Check sheet for the modelled part. Datum: model origin and axes. Units: mm. Face numbers are marked on the shaded views. A direction names the side the tool comes from. Round coordinates to 2 decimals unless told otherwise and drop trailing zeros. Loops run counter-clockwise (first coordinate to the right, second up) from the corner with the lowest first, then second, coordinate; pieces in that order, holes last. Notation, with made-up numbers: (-20, 34.5) -> (1, 34.5) arc R21 cw to (1, 73.5) -> close; hole circle Ø2 at (69, -10.75). An arc over 180 degrees is marked (long way). Return JSON: item names as keys, results as strings.
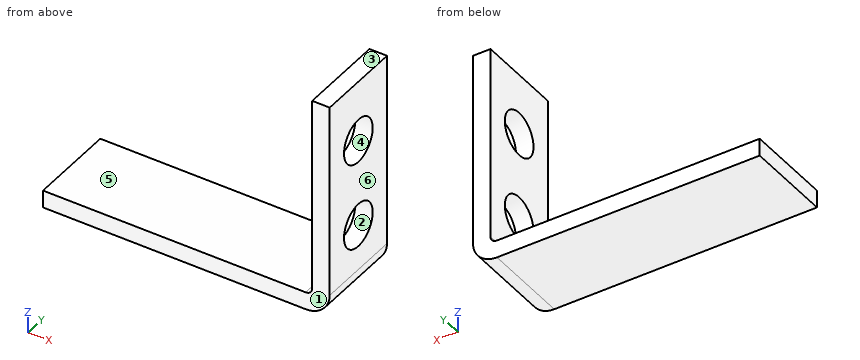
from build123d import *

# Parameters (mm, degrees)
SKETCH2_W          = 30
SKETCH2_H          = 10
BASE_FLANGE1_DEPTH = 2
EDGE_FLANGE1_DEPTH = 10
SKETCH10_R         = 2.5
CUT_EXTRUDE1_DEPTH = 39.713545169


# Sheet-metal steps are written as plain solids
with BuildPart() as part:
    # Sketch2 → Base-Flange1 (new body)
    with BuildSketch(Plane.XY):
        Rectangle(SKETCH2_W, SKETCH2_H)
    extrude(amount=-BASE_FLANGE1_DEPTH)

    # Edge-Flange1 section (across the edge) → Edge-Flange1 (add)
    with BuildSketch(Plane(origin=(15.7366, -5, 0), x_dir=(-1, 0, 0), z_dir=(0, 1, 0))):
        with BuildLine():
            Line((-2, 0.7366), (-2, 23))
            Line((-2, 23), (0, 23))
            Line((0, 23), (0, 0.7366))
            ThreePointArc((0, 0.7366), (0.215745145, 0.215745145), (0.7366, 0))
            Line((0.7366, 0), (0.7366, -2))
            ThreePointArc((0.7366, -2), (-1.198468417, -1.198468417), (-2, 0.7366))
        make_face()
    extrude(amount=EDGE_FLANGE1_DEPTH)

    # Sketch10 → Cut-Extrude1 (cut, through all)
    with BuildSketch(Plane.ZY.offset(-15.7366)):
        with Locations((6, 0)):
            Circle(SKETCH10_R)
        with Locations((16, 0)):
            Circle(SKETCH10_R)
    extrude(amount=-CUT_EXTRUDE1_DEPTH, mode=Mode.SUBTRACT)


solid = part.part
Q1. Go/stop test with flat-tipped pins: pin 1 (5 mm diameter, centred on y = -1, z = 8, fed in from -X); pin 2 (6 mm diameter, centred on y = 0, z = 6, fed in from +X); pin 3 (1.5 mm diameter, centred on x = 6.5, y = -1, fed in from +Z). Record where each tip stops, or that it passes through.
Results list:
{"pin 1": "x = 15.74", "pin 2": "x = 17.74", "pin 3": "z = 0"}
Q2. Section check A-A (z = 4). Record the boundary of the cut face in (x, y), then the cut area to 3 significant figures.
Results list:
{"outline": "(15.74, -5) -> (17.74, -5) -> (17.74, -1.5) -> (15.74, -1.5) -> close; (15.74, 1.5) -> (17.74, 1.5) -> (17.74, 5) -> (15.74, 5) -> close", "area": "14.0 mm^2"}
Q3. Section check C-C (y = -3). Record the boundary of the cut face in (x, z).
Results list:
{"outline": "(-15, -2) -> (15, -2) arc R2.74 ccw to (17.74, 0.74) -> (17.74, 23) -> (15.74, 23) -> (15.74, 0.74) arc R0.74 cw to (15, 0) -> (-15, 0) -> close"}
Q4. Draft check along Z on the marked faces 1, 2, 3 and 4. Enter one of: released by +Z, released by -Z, zero draft, split by the parting line, or undercut.
Results list:
{"face 1": "zero draft", "face 2": "undercut", "face 3": "released by +Z", "face 4": "undercut"}
Q5. Section check B-B (y = 0). Record the boundary of the cut face in (x, z).
Results list:
{"outline": "(-15, -2) -> (15, -2) arc R2.74 ccw to (17.74, 0.74) -> (17.74, 3.5) -> (15.74, 3.5) -> (15.74, 0.74) arc R0.74 cw to (15, 0) -> (-15, 0) -> close; (15.74, 8.5) -> (17.74, 8.5) -> (17.74, 13.5) -> (15.74, 13.5) -> close; (15.74, 18.5) -> (17.74, 18.5) -> (17.74, 23) -> (15.74, 23) -> close"}
Q6. Section check D-D (x = 4.5). Record the boundary of the cut face in (y, z), then the cut area to 3 significant figures.
Results list:
{"outline": "(-5, -2) -> (5, -2) -> (5, 0) -> (-5, 0) -> close", "area": "20.0 mm^2"}
Q7. Material ranges on line 1 (Y direction, x = 17.05, z = 6); line 2 (X direction, y = 2.5, z = 5.25); line 3 (Z direction, x = 5, y = -0.5), recorded low to high.
Results list:
{"line 1": "-5 to -2.5, 2.5 to 5", "line 2": "15.74 to 17.74", "line 3": "-2 to 0"}
Q8. Tool access check on the marked faces 5 and 6. Record the directions out of +Z, -Z, +X, -X, +Y, -Y that give a thin tool (end or side, any length) a straight path to the whole face; none if there is none.
Results list:
{"face 5": "+Z, -X, +Y, -Y", "face 6": "+Z, -Z, +X, +Y, -Y"}
